Check sheet for the modelled part. Datum: model origin and axes. Units: mm. A direction names the side the tool comes from. Coordinates: 2 decimals unless noted, no trailing zeros. Loops run counter-clockwise (first coordinate to the right, second up) from the corner with the lowest first, then second, coordinate; pieces in that order, holes last.
from build123d import *

# Parameters (mm, degrees)
ESQUISSE1_W                    = 85
ESQUISSE1_H                    = 55
BOSS_EXTRU_1_DEPTH             = 10
ESQUISSE2_W                    = 8
ESQUISSE2_H                    = 5
ESQUISSE2_W_2                  = 42
ENL_V_MAT_EXTRU_1_DEPTH        = 102.734949747
ESQUISSE3_R                    = 2
ENL_V_MAT_EXTRU_2_DEPTH        = 90.895772982
TROU_TARAUD_M3X0_51_AT_2_COUNT = 2
TROU_TARAUD_M3X0_51_AT_2_PITCH = 33
TROU_TARAUD_M3X0_51_AT_3_COUNT = 2
TROU_TARAUD_M3X0_51_AT_3_PITCH = 68
TROU_TARAUD_M3X0_52_D          = 2
TROU_TARAUD_M3X0_52_DEPTH      = 12
TROU_TARAUD_M3X0_52_TIP        = 0.600860619
ESQUISSE8_W                    = 28
ESQUISSE8_H                    = 10
ENL_V_MAT_EXTRU_3_DEPTH        = 102.734949747
ESQUISSE9_W                    = 6
ESQUISSE9_H                    = 30
ENL_V_MAT_EXTRU_4_DEPTH        = 90.895772982
CONG_1_R                       = 4


with BuildPart() as part:
    # Esquisse1 → Boss.-Extru.1 (new body)
    with BuildSketch(Plane.XY):
        with Locations((42.5, 0)):
            Rectangle(ESQUISSE1_W, ESQUISSE1_H)
    extrude(amount=BOSS_EXTRU_1_DEPTH)

    # Esquisse2 → Enlèv. mat.-Extru.1 (cut, through all)
    with BuildSketch(Plane(origin=(0, 27.5, 0), x_dir=(1, 0, 0), z_dir=(0, 1, 0))):
        with Locations((4, -2.5)):
            Rectangle(ESQUISSE2_W, ESQUISSE2_H)
        with Locations((54, -2.5)):
            Rectangle(ESQUISSE2_W_2, ESQUISSE2_H)
    extrude(amount=-ENL_V_MAT_EXTRU_1_DEPTH, mode=Mode.SUBTRACT)

    # Esquisse3 → Enlèv. mat.-Extru.2 (cut, through all)
    with BuildSketch(Plane.XY.offset(10)):
        with Locations((4, 0)):
            Circle(ESQUISSE3_R)
        with Locations((37, 0)):
            Circle(ESQUISSE3_R)
    extrude(amount=-ENL_V_MAT_EXTRU_2_DEPTH, mode=Mode.SUBTRACT)

    # Esquisse4 → Trou taraudé M3x0.51 (revolve, cut)
    with BuildSketch(Plane(origin=(4, -27.5, 7.5), x_dir=(0, 0, -1), z_dir=(1, 0, 0))):
        Polygon((0, 0), (0, 15.600860619), (1, 15), (1, 0), align=None)
    trou_taraud_m3x0_51 = revolve(axis=Axis((4, -33.85, 7.5), (0, 1, 0)), mode=Mode.SUBTRACT)

    # Trou taraudé M3x0.51 at 2: Trou taraudé M3x0.51 ×2
    with Locations(*[(i * TROU_TARAUD_M3X0_51_AT_2_PITCH, 0, 0) for i in range(1, TROU_TARAUD_M3X0_51_AT_2_COUNT)]):
        add(trou_taraud_m3x0_51, mode=Mode.SUBTRACT)

    # Trou taraudé M3x0.51 at 3: Trou taraudé M3x0.51 ×2
    with Locations(*[(i * TROU_TARAUD_M3X0_51_AT_3_PITCH, 0, 0) for i in range(1, TROU_TARAUD_M3X0_51_AT_3_COUNT)]):
        add(trou_taraud_m3x0_51, mode=Mode.SUBTRACT)

    # Symétrie1: Trou taraudé M3x0.51 across plane
    add(trou_taraud_m3x0_51.mirror(Plane.ZX), mode=Mode.SUBTRACT)

    # Symétrie1 copy 1 sketch → Symétrie1 copy 1 (revolve, cut)
    with BuildSketch(Plane(origin=(37, 27.5, 7.5), x_dir=(0, 0, -1), z_dir=(1, 0, 0))):
        Polygon((0, 0), (0, -15.600860619), (1, -15), (1, 0), align=None)
    revolve(axis=Axis((37, 33.85, 7.5), (0, 1, 0)), mode=Mode.SUBTRACT)

    # Symétrie1 copy 2 sketch → Symétrie1 copy 2 (revolve, cut)
    with BuildSketch(Plane(origin=(72, 27.5, 7.5), x_dir=(0, 0, -1), z_dir=(1, 0, 0))):
        Polygon((0, 0), (0, -15.600860619), (1, -15), (1, 0), align=None)
    revolve(axis=Axis((72, 33.85, 7.5), (0, 1, 0)), mode=Mode.SUBTRACT)

    # Trou taraudé M3x0.52
    with Locations(Plane(origin=(85, 0, 0), x_dir=(0, 0, -1), z_dir=(1, 0, 0))):
        with Locations((-5, 20), (-5, -20)):
            Hole(TROU_TARAUD_M3X0_52_D / 2, depth=TROU_TARAUD_M3X0_52_DEPTH)
            with Locations((0, 0, -(TROU_TARAUD_M3X0_52_DEPTH + TROU_TARAUD_M3X0_52_TIP / 2))):  # 118° drill point
                Cone(0, TROU_TARAUD_M3X0_52_D / 2, TROU_TARAUD_M3X0_52_TIP, mode=Mode.SUBTRACT)

    # Esquisse8 → Enlèv. mat.-Extru.3 (cut, through all)
    with BuildSketch(Plane.XZ.offset(27.5)):
        with Locations((14, 5)):
            Rectangle(ESQUISSE8_W, ESQUISSE8_H)
    extrude(amount=-ENL_V_MAT_EXTRU_3_DEPTH, mode=Mode.SUBTRACT)

    # Esquisse9 → Enlèv. mat.-Extru.4 (cut, through all)
    with BuildSketch(Plane.XY.offset(10)):
        with Locations((82, 0)):
            Rectangle(ESQUISSE9_W, ESQUISSE9_H)
    extrude(amount=-ENL_V_MAT_EXTRU_4_DEPTH, mode=Mode.SUBTRACT)

    # Congé1
    cong_1_edges = [part.edges().sort_by_distance(p)[0] for p in [
        (79, -15, 5),
        (79, 15, 5),
    ]]
    fillet(cong_1_edges, radius=CONG_1_R)


solid = part.part
(1) Set-up check for faces 4 (the face through (84, -15, 5)), 5 (the face through (72.89, -20.1, 7.04)), 6 (the face through (75, 0, 3)): record each of +Z, -Z, +X, -X, +Y, -Y from which the full face is reachable in a straight line by a thin tool's end or side.
(2) Draft check along Y on faces 1 (the face through (71.83, -12, 7.52)), 2 (the face through (54, 0, 5)), 3 (the face through (84, 15, 5)). Enter one of: pulls with the +Y half, pulls with the -Y half, needs draft (parallel to the pull), parting line crosses it, or undercut.
(3) Section check C-C, the plane y = 0. Enter the section's corners in (x, z), plus the area to 3 significant figures.
(4) Section check A-A, the plane y = 20. Enter the section's corners in (x, z), plus the area to 3 significant figures.
(5) Gauge pin test, flat ends, axial feed: P1, Ø6, axis at x = 60, y = -4, coming from the -Z side; P2, Ø3, axis at x = 54.5, z = 2.5, coming from the -Y side; P3, Ø1.8, axis at x = 37, z = 7.5, coming from the -Y side; P4, Ø1.6, axis at x = 37, z = 7.5, coming from the +Y side. Record the tip position at first contact, or that the pin passes through.
(6) Section check B-B, the plane z = 1.75. Enter the section's corners in (x, y), plus the area to 3 significant figures.
(7) Section check D-D, the plane y = -9. Enter the section's corners in (x, z), plus the area to 3 significant figures.
(8) Scan lines: line 1 along X through (y, z) = (24.25, 7.5); line 2 along X through (y, z) = (2, 4); line 3 along Z through (x, y) = (77, -20). Record each from-to range of solid material in increasing order.
Determined:
1. face 4: +Z, -Z, +X
1. face 5: -Y
1. face 6: -Z, +Y, -Y
2. face 1: pulls with the -Y half
2. face 2: needs draft
2. face 3: undercut
3. outline: (28, 0) - (33, 0) - (33, 5) - (35, 5) - (35, 10) - (28, 10) - close; (39, 5) - (75, 5) - (75, 0) - (79, 0) - (79, 10) - (39, 10) - close
3. area: 280 mm2
4. outline: (28, 0) - (33, 0) - (33, 5) - (72.4, 5) - (73, 6) - (85, 6) - (85, 10) - (28, 10) - close; (75, 0) - (85, 0) - (85, 4) - (75, 4) - close; hole circle Ø2 at (37, 7.5); hole circle Ø2 at (72, 7.5)
4. area: 331 mm2
5. P1: stops at z = 5
5. P2: passes through
5. P3: stops at y = -12.44
5. P4: stops at y = 12.38
6. outline: (28, -27.5) - (33, -27.5) - (33, 27.5) - (28, 27.5) - close; (75, -27.5) - (85, -27.5) - (85, -15) - (83, -15) arc R4 cw to (79, -11) - (79, 11) arc R4 cw to (83, 15) - (85, 15) - (85, 27.5) - (75, 27.5) - close
6. area: 652 mm2
7. outline: (28, 0) - (33, 0) - (33, 5) - (75, 5) - (75, 0) - (79, 0) - (79, 10) - (28, 10) - close
7. area: 300 mm2
8. line 1: x = 28 to 36, 38 to 71, 73 to 85
8. line 2: x = 28 to 33, 75 to 79
8. line 3: z = 0 to 4, 6 to 10
